Part model, mm, in its own coordinate system. A direction names the side the tool comes from. Give positions to 0.01 mm unless a question says otherwise; leave off trailing zeros. Write each loop counter-clockwise with the first axis right and the second up, starting at its lowest first coordinate (ties: lowest second). Pieces come first, ordered by that corner, then holes. Notation, with made-up numbers: M 62,28 L 94,28 A18 cw 94,54 Z; hole C 40,-29.5 d10. An arc over 180 degrees is marked long. Use CSV: the item, a comma, the result in double quotes. Start each with the question number.
Item 1: Drill centre lines: line 1 (Z direction, x = -50, y = 0); line 2 (X direction, y = 19, z = 11.5); line 3 (Y direction, x = 0, z = 4.5). Where is each one in solid material? Low to high. Write a range as [from, to].
Item 2: Pin check, flat tips, straight feed: pin 1 (13.5 mm diameter, centred on x = 0, y = 0, fed in from -Z); pin 2 (2 mm diameter, centred on y = -4.5, z = 4, fed in from +X); pin 3 (4 mm diameter, centred on x = 1.5, z = 4.5, fed in from -Y); pin 4 (1 mm diameter, centred on x = -46, z = 0.5, fed in from +Y). Stop position of each tip, or through.
Item 3: Cut at A-A (x = -5). Count the separate pieces of the cut face and the enclosed holes in it, then the cut area to 3 significant figures.
Item 4: Cut at B-B (x = -38.5). List the corners of the cut face in (y, z).
Item 5: Which spindle directions (+Z, -Z, +X, -X, +Y, -Y) get a long thin tool onto all of the face, cutting with end or side? Do faces 5 (the cylindrical face through (-37.72, -0.867, 1.345)), 6 (the flat face through (-5, 6, 10.5)), 7 (the flat face through (-7.253, 16.474, -2.425)). Say none if no direction does.
Item 6: Mould opens along Y. For faces 1 (the cylindrical face through (-14.18, 12.26, 13.15)), 2 (the cylindrical face through (-15.85, 33.15, -1.64)), 3 (the flat face through (2, -7.4, 9.5)), 4 (the cylindrical face through (-56.493, -1.517, 12.084)) say: released by +Y, released by -Y, zero draft, split by the parting line, or undercut.
from build123d import *

# Parameters (mm, degrees)
SZKIC1_R                         = 9.5
DODANIE_WYCI_GNI_CIE1_DEPTH      = 10.5
DODANIE_WYCI_GNI_CIE2_START      = -1
SZKIC4_R                         = 9.5
SZKIC4_R_2                       = 7.5
DODANIE_WYCI_GNI_CIE2_DEPTH      = 1
DODANIE_WYCI_GNI_CIE5_DEPTH      = 3.25
DODANIE_WYCI_GNI_CIE5_DEPTH_BACK = 13.75
ZAOKR_GLENIE1_R                  = 2
SFAZOWANIE1_SIZE                 = 0.5
ZAOKR_GLENIE2_R                  = 0.5
SFAZOWANIE2_SIZE                 = 1
OTWORY_USTALAJ_CE_8_0MM4_D       = 8
OTWORY_USTALAJ_CE_8_0MM4_DEPTH   = 40
OTWORY_USTALAJ_CE_8_0MM4_TIP     = 2.403442476110241
OTWORY_USTALAJ_CE_8_0MM2_D       = 8
OTWORY_USTALAJ_CE_8_0MM2_DEPTH   = 40
OTWORY_USTALAJ_CE_8_0MM2_TIP     = 2.403442476110241


with BuildPart() as part:
    # Szkic1 → Dodanie-wyciągnięcie1 (new body)
    with BuildSketch(Plane.XY):
        with BuildLine():
            Line((-18, -8.500000000000002), (-2.452989835267137, -11.746609760610767))
            ThreePointArc((-2.452989835267137, -11.746609760610767), (10.072083256378775, -6.523276697839391), (9.716034523496084, 7.042632543178169))
            Line((9.716034523496084, 7.042632543178169), (0.3948872336267733, 19.902112050551786))
            Line((0.3948872336267733, 19.902112050551786), (-15.118317795339578, 12.949380951965187))
            Line((-15.118317795339578, 12.949380951965187), (-14.300349430799978, 11.124298007380911))
            ThreePointArc((-14.300349430799978, 11.124298007380911), (-14.606664802217058, 9.460139845161555), (-16, 8.499999999999996))
            Line((-16, 8.499999999999996), (-18, 8.499999999999998))
            Line((-18, 8.499999999999998), (-18, -8.500000000000002))
        make_face()
        with Locations(Location((0, 0, 0), (0, 0, 180))):
            Circle(SZKIC1_R, mode=Mode.SUBTRACT)
    extrude(amount=DODANIE_WYCI_GNI_CIE1_DEPTH)

    # Szkic2 → Obrót1 (revolve)
    with BuildSketch(Plane.XY.offset(5.25), mode=Mode.PRIVATE) as obr_t1_sk:
        Polygon((-57.99999999999999, -6.94e-15), (-57.99999999999999, -7.000000000000007), (-55.99999999999999, -7.000000000000007), (-55.99999999999999, -6.950000000000007), (-18.000000000000004, -6.950000000000007), (-18, -2.2e-15), align=None)
    revolve(obr_t1_sk.sketch.rotate(Axis((0, 0, 5.25), (-1, -1.2e-16, 0)), 180), axis=Axis((0, 0, 5.25), (-1, -1.2e-16, 0)))

    # Szkic3 → Obrót2 (revolve)
    with BuildSketch(Plane.XY.offset(5.25)):
        Polygon((-23.721082571648417, 52.927405392943996), (-17.333292265603436, 55.79029466883262), (-16.515323901063837, 53.96521172424835), (-16.560950974678434, 53.94476251513487), (-1.0195520484260303, 19.26818656803362), (-7.361715280856409, 16.425746501258498), align=None)
    revolve(axis=Axis((0, 0, 5.25), (-0.4089841822698003, 0.9125414722921379, 0)))

    # Szkic4 → Dodanie-wyciągnięcie2 (add)
    with BuildSketch(Plane.XY.offset(10.5).offset(DODANIE_WYCI_GNI_CIE2_START)):
        with Locations(Location((0, 0, 0), (0, 0, 180))):
            Circle(SZKIC4_R)
        Circle(SZKIC4_R_2, mode=Mode.SUBTRACT)
    extrude(amount=DODANIE_WYCI_GNI_CIE2_DEPTH)

    # Szkic8 → Dodanie-wyciągnięcie5 (add, two sides: drawn at the far end of the back side and taken through both)
    with BuildSketch(Plane.XY.offset(10.5).offset(-DODANIE_WYCI_GNI_CIE5_DEPTH_BACK)):
        Polygon((-18, 8.499999999999998), (-18, -8.500000000000002), (-15.999999999999996, -8.917650689902482), (-16, 8.499999999999996), align=None)
        Polygon((1.5939791736338076, 18.247841631851692), (0.3948872336267733, 19.902112050551786), (-15.118317795339578, 12.949380951965187), (-14.300349430799978, 11.124298007380911), align=None)
    extrude(amount=DODANIE_WYCI_GNI_CIE5_DEPTH + DODANIE_WYCI_GNI_CIE5_DEPTH_BACK)

    # Zaokrąglenie1
    zaokr_glenie1_edges = [part.edges().sort_by_distance(p)[0] for p in [
        (-17, -8.708825344951242, -3.25),
        (-17, 8.499999999999996, -3.25),
        (-17, 8.499999999999996, 13.75),
        (-17, -8.708825344951242, 13.75),
        (0.9944332036302904, 19.07497684120174, -3.25),
        (-14.709333613069777, 12.036839479673048, -3.25),
        (-14.709333613069777, 12.036839479673048, 13.75),
        (0.9944332036302904, 19.07497684120174, 13.75),
    ]]
    fillet(zaokr_glenie1_edges, radius=ZAOKR_GLENIE1_R)

    # Sfazowanie1
    sfazowanie1_edges = [part.edges().sort_by_distance(p)[0] for p in [
        (5.655006848564945, 12.645237087514932, 0),
        (10.072083256378772, -6.523276697839393, 0),
        (-14.606664802217058, 9.460139845161555, 10.5),
        (10.072083256378772, -6.523276697839393, 10.5),
        (-9.226494917633566, -10.332130225256623, 0),
        (-9.226494917633566, -10.332130225256623, 10.5),
        (5.655006848564945, 12.645237087514932, 10.5),
        (-14.606664802217058, 9.460139845161555, 0),
    ]]
    chamfer(sfazowanie1_edges, length=SFAZOWANIE1_SIZE)

    # Zaokrąglenie2
    zaokr_glenie2_edges = [part.edges().sort_by_distance(p)[0] for p in [
        (9.5, -2.33e-15, 9.5),
    ]]
    fillet(zaokr_glenie2_edges, radius=ZAOKR_GLENIE2_R)

    # Sfazowanie2
    sfazowanie2_edges = [part.edges().sort_by_distance(p)[0] for p in [
        (-57.99999999999999, -7.000000000000007, 5.249999999999998),
        (-30.108872877693408, 50.06451611705539, 5.249999999999999),
    ]]
    chamfer(sfazowanie2_edges, length=SFAZOWANIE2_SIZE)

    # Otwory ustalające Ø8.0mm4
    with Locations(Plane(origin=(-23.721082572, 52.927405393, 5.25), x_dir=(0.912541472292, 0.40898418227, 0), z_dir=(-0.40898418227, 0.912541472292, 0))):
        with Locations((0, 0)):
            Hole(OTWORY_USTALAJ_CE_8_0MM4_D / 2, depth=OTWORY_USTALAJ_CE_8_0MM4_DEPTH)
            with Locations((0, 0, -(OTWORY_USTALAJ_CE_8_0MM4_DEPTH + OTWORY_USTALAJ_CE_8_0MM4_TIP / 2))):  # 118° drill point
                Cone(0, OTWORY_USTALAJ_CE_8_0MM4_D / 2, OTWORY_USTALAJ_CE_8_0MM4_TIP, mode=Mode.SUBTRACT)

    # Otwory ustalające Ø8.0mm2
    with Locations(Plane(origin=(-58, 0, 5.25), x_dir=(0, -1, 0), z_dir=(-1, 0, 0))):
        with Locations((0, 0)):
            Hole(OTWORY_USTALAJ_CE_8_0MM2_D / 2, depth=OTWORY_USTALAJ_CE_8_0MM2_DEPTH)
            with Locations((0, 0, -(OTWORY_USTALAJ_CE_8_0MM2_DEPTH + OTWORY_USTALAJ_CE_8_0MM2_TIP / 2))):  # 118° drill point
                Cone(0, OTWORY_USTALAJ_CE_8_0MM2_D / 2, OTWORY_USTALAJ_CE_8_0MM2_TIP, mode=Mode.SUBTRACT)


solid = part.part
Worked answers:
1,line 1,"z = [-1.7, 1.25], [9.25, 12.2]"
1,line 2,"x = [-11.85, -5.18], [-1.62, 1.05]"
1,line 3,"y = [-12, -9.5], [9.5, 19.73]"
2,pin 1,"passes through"
2,pin 2,"stops at x = 11.48"
2,pin 3,"stops at y = -12"
2,pin 4,"stops at y = 5.5"
3,separate pieces,"2"
3,enclosed holes,"1"
3,area,"231 mm^2"
4,outline,"C 0,5.25 d13.9; hole C 0,5.25 d8"
5,face 5,"-X"
5,face 6,"+Z, +X, -Y"
5,face 7,"none"
6,face 1,"released by -Y"
6,face 2,"undercut"
6,face 3,"undercut"
6,face 4,"split by the parting line"
